Geometry check sheet. Reference: the model listing, model coordinates, mm. A direction names the side the tool comes from. Round coordinates to 2 decimals unless told otherwise and drop trailing zeros. Write each loop counter-clockwise with the first axis right and the second up, starting at its lowest first coordinate (ties: lowest second). Pieces come first, ordered by that corner, then holes. Notation, with made-up numbers: (26, 15.25) -> (71, 15.25) arc R23 ccw to (71, 26.25) -> close; hole circle Ø10 at (4, 34). An arc over 180 degrees is marked (long way). Use a Markdown table: item, result.
Autodesk Inventor part; units mm, degrees
ref_plane "YZ Plane" through (0, 0, 0) normal (1, 0, 0) x (0, 1, 0)
ref_plane "XZ Plane" through (0, 0, 0) normal (0, 1, 0) x (-1, 0, 0)
ref_plane "XY Plane" through (0, 0, 0) normal (0, 0, 1) x (1, 0, 0)
sketch "Esquisse1" plane through (0, 0, 0) normal (0, 1, 0) x (-1, 0, 0)
  line L0 (0, 0) -> (8, 0)
  line L1 (8, 0) -> (8, -40)
  line L2 (8, -40) -> (0, -40)
  line L3 (0, -40) -> (0, 0)
  line L4 (0, 0) -> (8, 0)
  line L5 (8, 0) -> (8, 40)
  line L6 (8, 40) -> (0, 40)
  line L7 (0, 40) -> (0, 0)
  line L8 (0, 3.5) -> (-5, 3.5)
  line L9 (-5, 3.5) -> (-5, 0)
  line L10 (-5, 0) -> (0, 0)
  line L11 (0, 0) -> (0, 3.5)
  line L12 (-5, -3.5) -> (0, -3.5)
  line L13 (0, -3.5) -> (0, 0)
  line L14 (0, 0) -> (-5, 0)
  line L15 (-5, 0) -> (-5, -3.5)
  dimension "d0" = 40
  dimension "d1" = 40
  dimension "d2" = 8
  dimension "d3" = 8
  dimension "d4" = 3.5
  dimension "d5" = 3.5
  dimension "d6" = 5
  dimension "d7" = 5
extrude "Extrusion1" add sketch "Esquisse1" along normal blind 8
sketch "Esquisse2" plane through (0, 8, 0) normal (0, 1, 0) x (1, 0, 0)
  line L0 (4.25, 2.5) -> (1.25, 2.5)
  line L1 (1.25, 2.5) -> (1.25, -2.5)
  line L2 (1.25, -2.5) -> (4.25, -2.5)
  line L3 (4.25, -2.5) -> (4.25, 2.5)
  line L4 (0, 0) -> (3, 0)
  line L5 (3, -10) -> (3, 10)
  line L6 (1.25, -2.5) -> (4.25, 2.5)
  line L7 (4.25, 2.5) -> (1.25, 2.5)
  line L8 (4.25, -2.5) -> (1.25, 2.5)
  line L9 (-8, 40) -> (-8, -40)
  line L10 (0, 3.5) -> (0, 40)
  line L11 (0, 40) -> (-8, 40)
  line L12 (0, 40) -> (-8, 40)
  line L13 (-5.5, -39.9859) -> (-4, 40)
  line L14 (0, 0) -> (-4.75, 0.007)
  point P0 (4.25, 0)
  point P1 (2.75, 0)
  dimension "d7" = 5
  dimension "d15" = 0
  dimension "d10" = 5
  dimension "d11" = 3
  dimension "d33" = 40
  dimension "d34" = 2.5
  dimension "d35" = 7.5
extrude "Extrusion2" cut sketch "Esquisse2" against normal blind 7
fillet "Congé1" radius 0.1 1 edges at (1.25, 4.5, -2.5)
fillet "Congé2" radius 0.1 1 edges at (4.25, 4.5, -2.5)
fillet "Congé3" radius 0.1 1 edges at (4.25, 4.5, 2.5)
fillet "Congé4" radius 0.1 1 edges at (1.25, 4.5, 2.5)
properties part number "helicoptere"
(1) Section check A-A on y = 1.75. Record the cut outline in (x, z).
A:
| item | result |
|---|---|
| outline | (-8, -40) -> (0, -40) -> (0, -3.5) -> (5, -3.5) -> (5, 3.5) -> (0, 3.5) -> (0, 40) -> (-8, 40) -> close; hole (1.25, -2.4) arc R0.1 ccw to (1.35, -2.5) -> (4.15, -2.5) arc R0.1 ccw to (4.25, -2.4) -> (4.25, 2.4) arc R0.1 ccw to (4.15, 2.5) -> (1.35, 2.5) arc R0.1 ccw to (1.25, 2.4) -> close |
(2) Section check C-C on z = -25. Record the cut outline in (x, y), plus the area to 3 significant figures.
A:
| item | result |
|---|---|
| outline | (-8, 0) -> (0, 0) -> (0, 8) -> (-8, 8) -> close |
| area | 64.0 mm2 |
(3) Release check for a two-part mould opening along Z. For faces 4 (the face through (3, 4, -3.5)), 5 (the face through (1.25, 5, 0)), 6 (the face through (0, 4, 22)), 7 (the face through (2, 4, 3.5)) record: +Z half, -Z half, draft (parallel to the pull), parting line (faces both ways), or undercut.
A:
| item | result |
|---|---|
| face 4 | -Z half |
| face 5 | undercut |
| face 6 | draft |
| face 7 | +Z half |
(4) Section check B-B on z = -1. Record the cut outline in (x, y), plus the area to 3 significant figures.
A:
| item | result |
|---|---|
| outline | (-8, 0) -> (5, 0) -> (5, 8) -> (4.25, 8) -> (4.25, 1) -> (1.25, 1) -> (1.25, 8) -> (-8, 8) -> close |
| area | 83.0 mm2 |
(5) Gauge pin test, flat ends, axial feed: pin 1 Ø5 at (x, z) = (-0.5, -9.5) entering from -Y; pin 2 Ø2.5 at (y, z) = (4, 31) entering from +X; pin 3 Ø3 at (x, y) = (2.5, 3) entering from +Z; pin 4 Ø2 at (x, y) = (3.5, 4) entering from -Z. Record the tip position at first contact, or that the pin passes through.
A:
| item | result |
|---|---|
| pin 1 | stops at y = 0 |
| pin 2 | stops at x = 0 |
| pin 3 | stops at z = 3.5 |
| pin 4 | stops at z = -3.5 |
(6) Thickness scan on line 1 (X direction, y = 7.25, z = 0); line 2 (Z direction, x = 3, y = 6.75); line 3 (X direction, y = 0.5, z = -10). Record the ranges inside material, lowest first.
A:
| item | result |
|---|---|
| line 1 | x = -8 to 1.25, 4.25 to 5 |
| line 2 | z = -3.5 to -2.5, 2.5 to 3.5 |
| line 3 | x = -8 to 0 |
(7) Access from +Z, -Z, +X, -X, +Y, -Y to the whole of each face (thin tool, end or side, straight path). Record for faces 1 (the face through (3, 1, 0)), 2 (the face through (0, 4, -22)), 3 (the face through (-4, 4, 40)).
A:
| item | result |
|---|---|
| face 1 | +Y |
| face 2 | -Z, +X, +Y, -Y |
| face 3 | +Z, +X, -X, +Y, -Y |
